The drawing under review shows one solid part. Ordinate dimensions are in mm from its lowest x, y, z. A direction names the side the tool comes from. Round coordinates to 2 decimals unless told otherwise and drop trailing zeros. Order: outer loops, then holes, each group sorted by start corner. A loop starts at its lowest first (then second) coordinate and runs counter-clockwise, first axis right, second up. Notation, with made-up numbers: M 8,-26.5 L 49,-26.5 A20 ccw 49,3.5 Z; hole C 89.25,-20.5 d5. An arc over 180 degrees is marked long. Use a Markdown table: item, result.
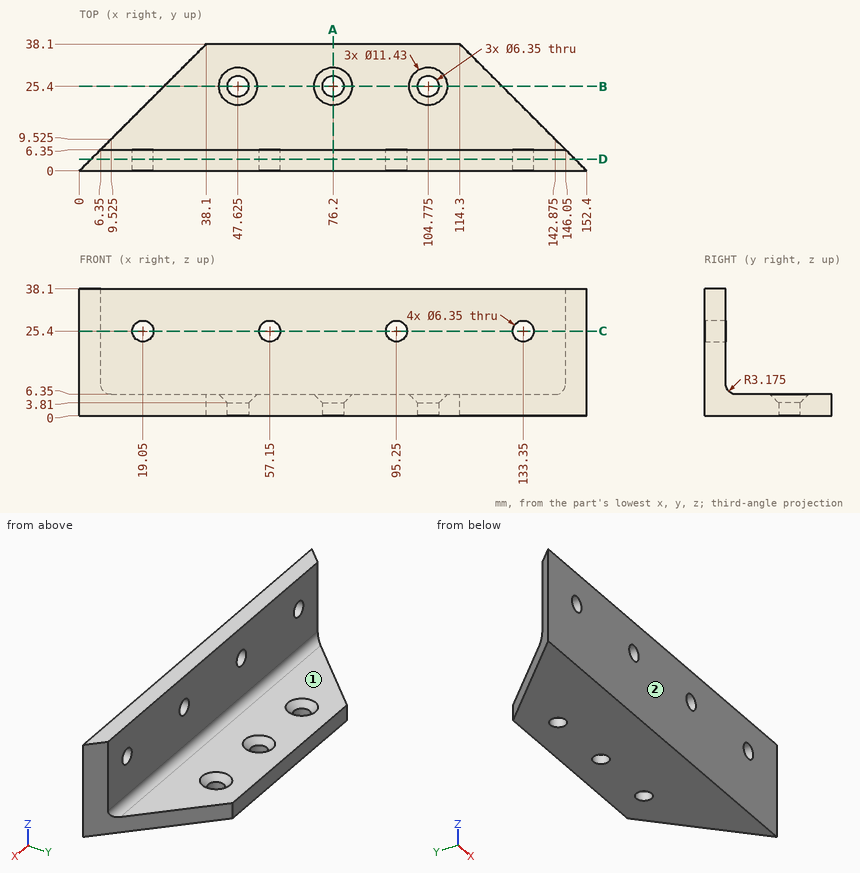
Q1. Add section A-A (x = 76.2). Write out the cut boundary in (y, z) (3 decimals), then the cut area to 3 significant figures.
Determined:
| item | result |
|---|---|
| outline | M 0,0 L 22.225,0 L 22.225,3.81 L 19.685,6.35 L 9.525,6.35 A3.175 cw 6.35,9.525 L 6.35,38.1 L 0,38.1 Z; M 28.575,0 L 38.1,0 L 38.1,6.35 L 31.115,6.35 L 28.575,3.81 Z |
| area | 399 mm^2 |
Q2. Machinability: for the marked faces 1 and 2, which of the approach directions +Z, -Z, +X, -X, +Y, -Y give a long, thin tool a straight path to every point of the face, cutting with its end or side? Answer none if there is none.
Determined:
| item | result |
|---|---|
| face 1 | +Z, +X, -X, +Y |
| face 2 | +Z, -Z, +X, -X, -Y |
Q3. Add section D-D (y = 3.5). Write out the cut boundary in (x, z) (3 decimals), then the cut area to 3 significant figures.
Determined:
| item | result |
|---|---|
| outline | M 3.5,0 L 148.9,0 L 148.9,38.1 L 3.5,38.1 Z; hole C 19.05,25.4 d6.35; hole C 57.15,25.4 d6.35; hole C 95.25,25.4 d6.35; hole C 133.35,25.4 d6.35 |
| area | 5,410 mm^2 |
Q4. Clearance check with flat-ended pins moving along their axes: pin 1 (10 mm diameter, centred on x = 47.625, y = 25.4, fed in from +Z) (3 decimals); pin 2 (12 mm diameter, centred on x = 123, y = 21.5, fed in from +Z); pin 3 (10 mm diameter, centred on y = 7.5, z = 33, fed in from -X). State where each tip first meets the part, or that it passes through.
Determined:
| item | result |
|---|---|
| pin 1 | stops at z = 5.635 |
| pin 2 | stops at z = 6.35 |
| pin 3 | stops at x = 2.5 |
Q5. Add section B-B (y = 25.4). Write out the cut boundary in (x, z) (3 decimals).
Determined:
| item | result |
|---|---|
| outline | M 25.4,0 L 44.45,0 L 44.45,3.81 L 41.91,6.35 L 25.4,6.35 Z; M 50.8,0 L 73.025,0 L 73.025,3.81 L 70.485,6.35 L 53.34,6.35 L 50.8,3.81 Z; M 79.375,0 L 101.6,0 L 101.6,3.81 L 99.06,6.35 L 81.915,6.35 L 79.375,3.81 Z; M 107.95,0 L 127,0 L 127,6.35 L 110.49,6.35 L 107.95,3.81 Z |
Q6. Wall thickness on line 1 along X through (y, z) = (4.75, 25.4) (3 decimals); line 2 along Z through (x, y) = (19, 3); line 3 along Y through (x, z) = (104, 34): over which ranges is each line inside the solid? List them lowest first. Write a range as [from, to].
Determined:
| item | result |
|---|---|
| line 1 | x = [4.75, 15.875], [22.225, 53.975], [60.325, 92.075], [98.425, 130.175], [136.525, 147.65] |
| line 2 | z = [0, 22.23], [28.57, 38.1] |
| line 3 | y = [0, 6.35] |
Q7. Add section C-C (z = 25.4). Write out the cut boundary in (x, y) (3 decimals), then the cut area to 3 significant figures.
Determined:
| item | result |
|---|---|
| outline | M 0,0 L 15.875,0 L 15.875,6.35 L 6.35,6.35 Z; M 22.225,0 L 53.975,0 L 53.975,6.35 L 22.225,6.35 Z; M 60.325,0 L 92.075,0 L 92.075,6.35 L 60.325,6.35 Z; M 98.425,0 L 130.175,0 L 130.175,6.35 L 98.425,6.35 Z; M 136.525,0 L 152.4,0 L 146.05,6.35 L 136.525,6.35 Z |
| area | 766 mm^2 |
